```python
from build123d import *

# Parameters (mm, degrees)
BOSS_EXTRUDE1_START  = -82.5
BOSS_EXTRUDE1_DEPTH  = 82.5
SKETCH2_W            = 8.569638255
SKETCH2_H            = 10
SKETCH2_H_2          = 18.5
CUT_EXTRUDE1_DEPTH   = 93.549500309
FILLET2_R            = 2
FILLET3_R            = 0.5
CUT_EXTRUDE2_START   = -17.5
SKETCH2_3_W          = 11.636747081
SKETCH2_3_H          = 15
CUT_EXTRUDE2_DEPTH   = 76.049500309
FILLET1_R            = 1.5
BOSS_EXTRUDE3_START  = -3.5
BOSS_EXTRUDE3_DEPTH  = 3
BOSS_EXTRUDE4_START  = -5
BOSS_EXTRUDE4_DEPTH  = 1.5
FILLET5_R            = 0.5
FILLET5_OF_MIRROR4_R = 0.5


# Read off the part's stored shape, not the designer's step: Boss-Extrude1
with BuildPart() as part:
    # Boss-Extrude1 outline → Boss-Extrude1 (new body)
    with BuildSketch(Plane.XY.offset(-2).offset(BOSS_EXTRUDE1_START)):
        Polygon((17.868316672, 32.1), (17.868316672, 29.85), (15.868316672, 29.85), (15.868316672, 30.024283949), (9.5, 30.024283949), (9.5, 28.024283949), (14, 28), (14, 27.85), (17.868316672, 27.85), (17.868316672, 0), (19.868316672, 0), (19.868316672, 32.1), align=None)
    boss_extrude1 = extrude(amount=BOSS_EXTRUDE1_DEPTH)

    # Mirror1: Boss-Extrude1 across plane
    add(boss_extrude1.mirror(Plane.ZX))

    # Sketch2 → Cut-Extrude1 (cut, through all)
    with BuildSketch(Plane(origin=(0, 0, 0), x_dir=(1, 0, 0), z_dir=(0, 1, 0))):
        with Locations((8.715180872, 16.2)):
            Rectangle(SKETCH2_W, SKETCH2_H)
        with Locations((8.715180872, 37)):
            Rectangle(SKETCH2_W, SKETCH2_H_2)
    extrude(amount=CUT_EXTRUDE1_DEPTH, mode=Mode.SUBTRACT)

    # Fillet2
    fillet2_edges = [part.edges().sort_by_distance(p)[0] for p in [
        (17.868316672, 27.85, -43.25),
        (17.868316672, -27.85, -43.25),
    ]]
    fillet(fillet2_edges, radius=FILLET2_R)

    # Fillet3
    # the kernel refuses this fillet: 0.5 mm, written as the material it adds along each edge
    with BuildSketch(Plane(origin=(15.868316672, -29.85, -84.5), x_dir=(0, -1, 0), z_dir=(0, 0, 1))) as fillet3_piece_1:
        with BuildLine():
            CenterArc((0.5, 0.379353469), FILLET3_R, 180, 49.350336553)
            Line((0, 0.379353469), (-0.01, 0.379353469))
            Line((-0.01, 0.379353469), (-0.01, 0))
            Line((-0.01, 0), (0, -0.01))
            ThreePointArc((0, -0.01), (0.087141974, -0.01), (0.167769628, -0.007587069))
            Line((0.167769628, -0.007587069), (0.174283949, 0))
        make_face()
    extrude(amount=82.5)
    with BuildSketch(Plane(origin=(17.868316672, -29.85, -84.5), x_dir=(-1, 0, 0), z_dir=(0, 0, 1))) as fillet3_piece_2:
        with BuildLine():
            CenterArc((FILLET3_R, FILLET3_R), FILLET3_R, 180, 90)
            Line((0, FILLET3_R), (-FILLET3_R * 0.02, FILLET3_R))
            Line((-FILLET3_R * 0.02, FILLET3_R), (-FILLET3_R * 0.02, -FILLET3_R * 0.02))
            Line((-FILLET3_R * 0.02, -FILLET3_R * 0.02), (FILLET3_R, -FILLET3_R * 0.02))
            Line((FILLET3_R, -FILLET3_R * 0.02), (FILLET3_R, 0))
        make_face()
    extrude(amount=82.5)
    with BuildSketch(Plane(origin=(17.868316672, 29.85, -84.5), x_dir=(-1, 0, 0), z_dir=(0, 0, 1))) as fillet3_piece_3:
        with BuildLine():
            CenterArc((FILLET3_R, -FILLET3_R), FILLET3_R, 90, 90)
            Line((0, -FILLET3_R), (-FILLET3_R * 0.02, -FILLET3_R))
            Line((-FILLET3_R * 0.02, -FILLET3_R), (-FILLET3_R * 0.02, FILLET3_R * 0.02))
            Line((-FILLET3_R * 0.02, FILLET3_R * 0.02), (FILLET3_R, FILLET3_R * 0.02))
            Line((FILLET3_R, FILLET3_R * 0.02), (FILLET3_R, 0))
        make_face()
    extrude(amount=82.5)
    with BuildSketch(Plane(origin=(15.868316672, 29.85, -84.5), x_dir=(0, 1, 0), z_dir=(0, 0, 1))) as fillet3_piece_4:
        with BuildLine():
            CenterArc((0.5, -0.379353469), FILLET3_R, 130.649663447, 49.350336553)
            Line((0, -0.379353469), (-0.01, -0.379353469))
            Line((-0.01, -0.379353469), (-0.01, 0))
            Line((-0.01, 0), (0, 0.01))
            ThreePointArc((0, 0.01), (0.087141974, 0.01), (0.167769628, 0.007587069))
            Line((0.167769628, 0.007587069), (0.174283949, 0))
        make_face()
    extrude(amount=82.5)

    # Sketch2<3> → Cut-Extrude2 (cut, through all)
    with BuildSketch(Plane(origin=(0, 0, 0), x_dir=(1, 0, 0), z_dir=(0, 1, 0)).offset(CUT_EXTRUDE2_START)):
        with Locations((19.818373541, 53.901910681)):
            Rectangle(SKETCH2_3_W, SKETCH2_3_H)
    extrude(amount=-CUT_EXTRUDE2_DEPTH, mode=Mode.SUBTRACT)

    # Fillet1
    fillet1_edges = [part.edges().sort_by_distance(p)[0] for p in [
        (18.868316672, -17.5, -46.401910681),
        (14, -29.012141975, -46.401910681),
        (14, -29.012141975, -61.401910681),
        (18.868316672, -17.5, -61.401910681),
        (13, 29.014840191, -11.2),
        (13, 29.014840191, -21.2),
        (13, 29.014840191, -27.75),
        (13, 29.014840191, -46.25),
    ]]
    fillet(fillet1_edges, radius=FILLET1_R)

    # Sketch3 → Boss-Extrude3 (add)
    with BuildSketch(Plane.XY.offset(BOSS_EXTRUDE3_START)):
        Polygon((11.5, 28.013491083), (13, 28.005396433), (13, 25.013491083), (11.5, 25.013491083), align=None)
    boss_extrude3 = extrude(amount=-BOSS_EXTRUDE3_DEPTH)

    # Sketch3<6> → Boss-Extrude4 (add)
    with BuildSketch(Plane.XY.offset(BOSS_EXTRUDE4_START)):
        Polygon((13, 28.005396433), (17.868316672, 27.979124888), (17.868316672, 25.013491083), (13, 25.013491083), align=None)
    boss_extrude4 = extrude(amount=BOSS_EXTRUDE4_DEPTH)

    # Fillet5
    fillet5_edges = [part.edges().sort_by_distance(p)[0] for p in [
        (11.5, 26.513491083, -3.5),
    ]]
    fillet(fillet5_edges, radius=FILLET5_R)

    # Mirror4: Boss-Extrude3, Boss-Extrude4 across plane
    add(boss_extrude3.mirror(Plane.ZX))
    add(boss_extrude4.mirror(Plane.ZX))

    # Fillet5 of Mirror4
    fillet5_of_mirror4_edges = [part.edges().sort_by_distance(p)[0] for p in [
        (11.5, -26.513491083, -3.5),
    ]]
    fillet(fillet5_of_mirror4_edges, radius=FILLET5_OF_MIRROR4_R)


solid = part.part
```
Geometry: final body of the model. Coordinates: model frame, mm. A direction names the side the tool comes from. Round coordinates to 2 decimals unless told otherwise and drop trailing zeros. Write each loop counter-clockwise with the first axis right and the second up, starting at its lowest first coordinate (ties: lowest second). Pieces come first, ordered by that corner, then holes.
Item 1: Pin query (flat end, axial travel): P1, Ø0.6, axis at y = 29, z = -38.5, coming from the -X side; P2, Ø0.6, axis at x = 15.5, z = -62, coming from the -Y side; P3, Ø2, axis at x = 19, z = -56.5, coming from the -Y side. Return the tip coordinate at first contact, or that it passes through.
Item 2: Mould query, pull axis Z, two halves, no side actions, for faces 4 (the face through (18, -27, -61.402)), 5 (the face through (17.298, 27.249, -44.194)), 6 (the face through (18.1, 0.4, -2)). Classes: +Z half, -Z half, draft (parallel to the pull), parting line (faces both ways), or undercut.
Item 3: Material intervals for L1, parallel to Y at x = 14.5, z = -22; L2, parallel to Y at x = 12, z = -73; L3, parallel to X at y = 18, z = -70, sorted ascending.
Item 4: Section query B-B (x = 18.75). Return loops of the section in (y, z), plus the area to 3 significant figures.
Item 5: Set-up query: faces 1 (the face through (10, 29, -21.2)), 2 (the face through (17.298, 27.249, -2.74)), 3 (the face through (14, -25.013, -4)). Return all of +Z, -Z, +X, -X, +Y, -Y with unobstructed straight access to the full face (end or side cutting, diameter ignored); none if empty.
Item 6: Section query C-C (y = -1.5). Return loops of the section in (x, z), plus the area to 3 significant figures.
Item 7: Section query A-A (z = -31). Return loops of the section in (x, y).
Completed:
1. P1: stops at x = 13
1. P2: stops at y = -30.02
1. P3: stops at y = -17.5
2. face 4: undercut
2. face 5: draft
2. face 6: +Z half
3. L1: y = -30.02 to -27.85, 27.85 to 30.02
3. L2: y = -30.02 to -28.01, 28.01 to 30.02
3. L3: x = 17.87 to 19.87
4. outline: (-32.1, -84.5) - (32.1, -84.5) - (32.1, -2) - (-32.1, -2) - (-32.1, -46.4) - (-19, -46.4) arc R1.5 cw to (-17.5, -47.9) - (-17.5, -59.9) arc R1.5 cw to (-19, -61.4) - (-32.1, -61.4) - close
4. area: 5,080 mm2
5. face 1: -X, +Y
5. face 2: +Z, -X
5. face 3: +Z, -Z, -X
6. outline: (17.87, -84.5) - (19.87, -84.5) - (19.87, -2) - (17.87, -2) - close
6. area: 165 mm2
7. outline: (9.5, -30.02) - (15.87, -30.02) arc R0.5 cw to (16.25, -29.85) - (17.37, -29.85) arc R0.5 cw to (17.87, -30.35) - (17.87, -32.1) - (19.87, -32.1) - (19.87, 32.1) - (17.87, 32.1) - (17.87, 30.35) arc R0.5 cw to (17.37, 29.85) - (16.25, 29.85) arc R0.5 cw to (15.87, 30.02) - (13, 30.02) - (13, 28.01) - (14, 28) - (14, 27.85) - (15.87, 27.85) arc R2 cw to (17.87, 25.85) - (17.87, -25.85) arc R2 cw to (15.87, -27.85) - (14, -27.85) - (14, -28) - (9.5, -28.02) - close
